Verification items for the finished model (mm, model axes). A direction names the side the tool comes from. Coordinates: 2 decimals unless noted, no trailing zeros. Write each loop counter-clockwise with the first axis right and the second up, starting at its lowest first coordinate (ties: lowest second). Pieces come first, ordered by that corner, then holes. Notation, with made-up numbers: M -31,57 L -21,57 A13 cw -21,75 Z; hole C 72.5,25 d5. An arc over 180 degrees is marked long. One line per item, written item: value.
```python
from build123d import *

# Parameters (mm, degrees)
SKETCH010_R     = 1.1
PAD006_DEPTH    = 2
SKETCH011_W     = 2
SKETCH011_H     = 16.6
SKETCH011_W_2   = 27.6
SKETCH011_H_2   = 2
PAD007_DEPTH    = 1.6
SKETCH012_R     = 1.9
SKETCH012_R_2   = 4.3
SKETCH012_R_3   = 1.65
PAD008_DEPTH    = 2
SKETCH013_W     = 6
SKETCH013_H     = 6.6
SKETCH013_W_2   = 3.5
SKETCH013_H_2   = 4
POCKET002_DEPTH = 1.5


with BuildPart() as part:
    # Sketch010 → Pad006 (new body)
    with BuildSketch(Plane.XY.offset(4.8)):
        with BuildLine():
            Line((-25, -17), (25, -17))
            ThreePointArc((25, -17), (26.414214, -16.414214), (27, -15))
            Line((27, -15), (27, 15))
            ThreePointArc((27, 15), (26.414214, 16.414214), (25, 17))
            Line((25, 17), (-25, 17))
            ThreePointArc((-25, 17), (-26.414214, 16.414214), (-27, 15))
            Line((-27, 15), (-27, -15))
            ThreePointArc((-27, -15), (-26.414214, -16.414214), (-25, -17))
        make_face()
        with Locations((-22, 12)):
            Circle(SKETCH010_R, mode=Mode.SUBTRACT)
        with Locations((22, 12)):
            Circle(SKETCH010_R, mode=Mode.SUBTRACT)
        with Locations((-22, -12)):
            Circle(SKETCH010_R, mode=Mode.SUBTRACT)
        with Locations((22, -12)):
            Circle(SKETCH010_R, mode=Mode.SUBTRACT)
        with BuildLine():
            Line((-18.5, -15), (18.5, -15))
            ThreePointArc((25, -8.5), (20.403806, -10.403806), (18.5, -15))
            Line((25, -8.5), (25, 8.5))
            ThreePointArc((18.5, 15), (20.403806, 10.403806), (25, 8.5))
            Line((18.5, 15), (-18.5, 15))
            ThreePointArc((-25, 8.5), (-20.403806, 10.403806), (-18.5, 15))
            Line((-25, 8.5), (-25, -8.5))
            ThreePointArc((-18.5, -15), (-20.403806, -10.403806), (-25, -8.5))
        make_face(mode=Mode.SUBTRACT)
    extrude(amount=PAD006_DEPTH)

    # Sketch011 (on Face21 of Pad006) → Pad007 (join)
    with BuildSketch(Plane(origin=(0, 0, 4.8), x_dir=(1, 0, 0), z_dir=(0, 0, -1))):
        with Locations((-26, 0)):
            Rectangle(SKETCH011_W, SKETCH011_H)
        with Locations((26, 0)):
            Rectangle(SKETCH011_W, SKETCH011_H)
        with Locations((0, 16)):
            Rectangle(SKETCH011_W_2, SKETCH011_H_2)
    extrude(amount=PAD007_DEPTH)

    # Sketch012 (on Face3 of Pad007) → Pad008 (join)
    with BuildSketch(Plane.XY.offset(6.8)):
        with BuildLine():
            Line((-25, -17), (25, -17))
            ThreePointArc((25, -17), (26.414214, -16.414214), (27, -15))
            Line((27, -15), (27, 15))
            ThreePointArc((27, 15), (26.414214, 16.414214), (25, 17))
            Line((25, 17), (-25, 17))
            ThreePointArc((-25, 17), (-26.414214, 16.414214), (-27, 15))
            Line((-27, 15), (-27, -15))
            ThreePointArc((-27, -15), (-26.414214, -16.414214), (-25, -17))
        make_face()
        with Locations((-22, 12)):
            Circle(SKETCH012_R, mode=Mode.SUBTRACT)
        with Locations((22, 12)):
            Circle(SKETCH012_R, mode=Mode.SUBTRACT)
        with Locations((-22, -12)):
            Circle(SKETCH012_R, mode=Mode.SUBTRACT)
        with Locations((22, -12)):
            Circle(SKETCH012_R, mode=Mode.SUBTRACT)
        with Locations((0, 2)):
            Circle(SKETCH012_R_2, mode=Mode.SUBTRACT)
        with Locations((-18, -3.6)):
            Circle(SKETCH012_R_3, mode=Mode.SUBTRACT)
    extrude(amount=PAD008_DEPTH)

    # Sketch013 (on Face24 of Pad008) → Pocket002 (cut)
    with BuildSketch(Plane(origin=(0, 0, 6.8), x_dir=(1, 0, 0), z_dir=(0, 0, -1))):
        with Locations((-18, 3.6)):
            Rectangle(SKETCH013_W, SKETCH013_H)
        with Locations((-7, -5)):
            Rectangle(SKETCH013_W_2, SKETCH013_H_2)
        with Locations((-7, 1)):
            Rectangle(SKETCH013_W_2, SKETCH013_H_2)
        with Locations((7, -5)):
            Rectangle(SKETCH013_W_2, SKETCH013_H_2)
        with Locations((7, 1)):
            Rectangle(SKETCH013_W_2, SKETCH013_H_2)
        with Locations((-15, 10)):
            Rectangle(SKETCH013_W_2, SKETCH013_H_2)
    extrude(amount=-POCKET002_DEPTH, mode=Mode.SUBTRACT)


solid = part.part
```
Item 1: Scan lines: line 1 (Y direction, x = 22, z = 7.8); line 2 (X direction, y = 4.5, z = 8); line 3 (Y direction, x = -22, z = 5.4). Record each from-to range of solid material in increasing order.
The answers:
line 1: y = -17 to -13.9, -10.1 to 10.1, 13.9 to 17
line 2: x = -27 to -8.75, -5.25 to -3.5, 3.5 to 5.25, 8.75 to 27
line 3: y = -17 to -13.1, -10.9 to -9.23, 9.23 to 10.9, 13.1 to 17
Item 2: Cross-section at A-A, the plane z = 3.9. Enter the section's corners in (x, y), and give its area (3 significant figures).
The answers:
outline: M -27,-8.3 L -25,-8.3 L -25,8.3 L -27,8.3 Z; M -13.8,-17 L 13.8,-17 L 13.8,-15 L -13.8,-15 Z; M 25,-8.3 L 27,-8.3 L 27,8.3 L 25,8.3 Z
area: 122 mm²
Item 3: Cross-section at B-B, the plane y = 2. Enter the section's corners in (x, z), and give its area (3 significant figures).
The answers:
outline: M -27,3.2 L -25,3.2 L -25,6.8 L -4.3,6.8 L -4.3,8.8 L -27,8.8 Z; M 4.3,6.8 L 25,6.8 L 25,3.2 L 27,3.2 L 27,8.8 L 4.3,8.8 Z
area: 105 mm²
Item 4: Cross-section at D-D, the plane x = 22. Enter the section's corners in (y, z), and give its area (3 significant figures).
The answers:
outline: M -17,4.8 L -13.1,4.8 L -13.1,6.8 L -13.9,6.8 L -13.9,8.8 L -17,8.8 Z; M -10.9,4.8 L -9.23,4.8 L -9.23,6.8 L 9.23,6.8 L 9.23,4.8 L 10.9,4.8 L 10.9,6.8 L 10.1,6.8 L 10.1,8.8 L -10.1,8.8 L -10.1,6.8 L -10.9,6.8 Z; M 13.1,4.8 L 17,4.8 L 17,8.8 L 13.9,8.8 L 13.9,6.8 L 13.1,6.8 Z
area: 75.1 mm²
Item 5: Cross-section at C-C, the plane x = -12.5. Enter the section's corners in (y, z).
The answers:
outline: M -17,3.2 L -15,3.2 L -15,6.8 L 15,6.8 L 15,4.8 L 17,4.8 L 17,8.8 L -17,8.8 Z
Item 6: Go/stop test with flat-tipped pins: P1, Ø3, axis at x = 7.5, y = -1, coming from the -Z side; P2, Ø1.3, axis at y = -16.5, z = 4, coming from the +X side; P3, Ø2.5, axis at x = -22, y = -12, coming from the -Z side; P4, Ø3, axis at x = 22.5, y = -12.5, coming from the +Z side. Record where each tip stops, or that it passes through.
The answers:
P1: stops at z = 6.8
P2: stops at x = 13.8
P3: stops at z = 4.8
P4: stops at z = 8.8
Item 7: Draft check along X on faces 4 (the face through (26.4, -16.43, 6.77)), 5 (the face through (8.75, -1, 8)), 6 (the face through (26, 8.3, 4)), 7 (the face through (-26.4, 16.43, 6.77)). Enter one of: released by +X, released by -X, zero draft, split by the parting line, or undercut.
The answers:
face 4: released by +X
face 5: undercut
face 6: zero draft
face 7: released by -X
Item 8: Access from +Z, -Z, +X, -X, +Y, -Y to the whole of each face (thin tool, end or side, straight path). Record for faces 1 (the face through (-19.31, -4.6, 8.55)), 2 (the face through (-15, -8, 8)), 3 (the face through (-23.508, -13.156, 7.786)).
The answers:
face 1: +Z, -Z
face 2: -Z
face 3: +Z
